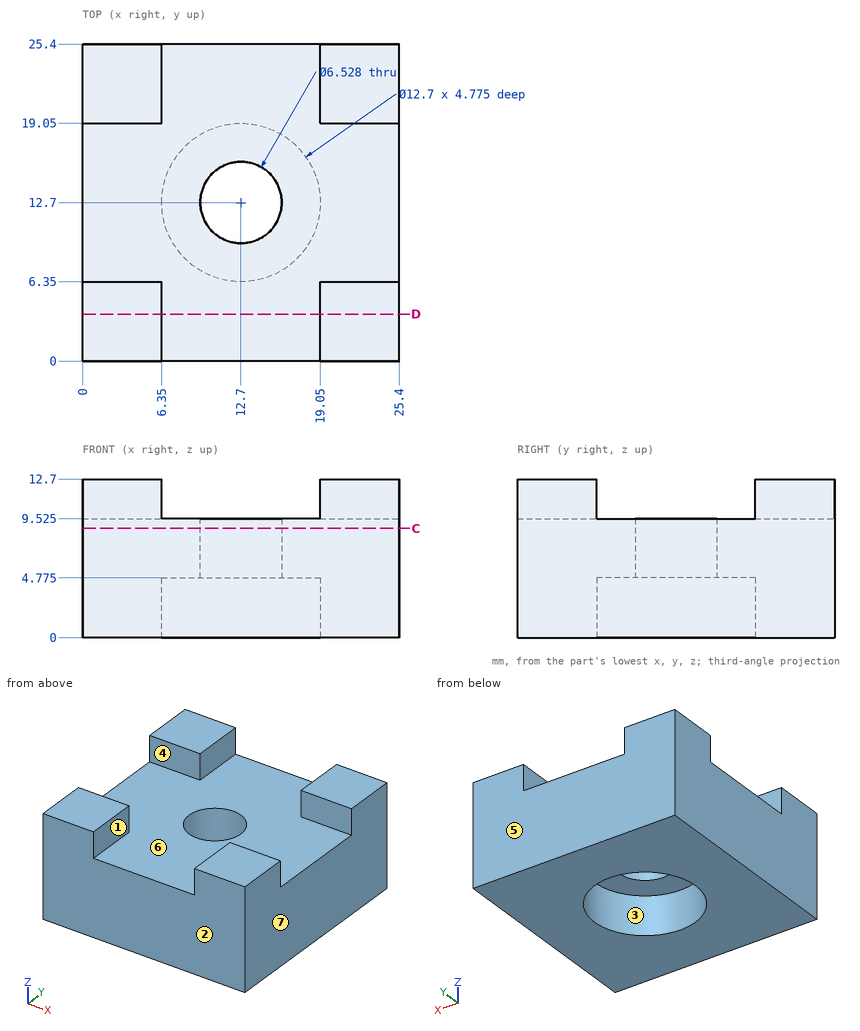
Drawing for the job (mm, zero at the part's lowest x, y, z). A direction names the side the tool comes from. Round coordinates to 2 decimals unless told otherwise and drop trailing zeros. Loops run counter-clockwise (first coordinate to the right, second up) from the corner with the lowest first, then second, coordinate; pieces in that order, holes last. Notation, with made-up numbers: (49.25, -31.5) - (91.25, -31.5) arc R24 cw to (91.25, -2.5) - close; hole circle Ø2 at (44, -10). An arc over 180 degrees is marked (long way). Return JSON: item names as keys, results as strings. Group by question number.
Q1. Tool access for the marked faces 1, 2, 3 and 4: list every direction of +Z, -Z, +X, -X, +Y, -Y with a clear straight run to the whole face (end or side of a thin tool).
Q2. Drill centre lines: line 1 along Y through (x, z) = (12.7, 6.15); line 2 along Y through (x, z) = (12.7, 3.6); line 3 along Z through (x, y) = (16.5, 18.75) (3 decimals). Where is each one in solid material? Low to high. Write a range as [from, to].
Q3. Flat gauge pins, fed straight in: pin 1 Ø7.5 at (x, y) = (12.7, 12.7) entering from +Z (3 decimals); pin 2 Ø4 at (x, y) = (14.5, 12) entering from -Z (3 decimals). Where does each tip first touch, or does it go through?
Q4. Two-plate mould, pull along Y, no slides. Class the marked faces 5, 6 and 7: +Y half, -Y half, draft (parallel to the pull), parting line (faces both ways), or undercut.
Q5. Band-saw the part on D-D on y = 3.75. Give the cut face in (x, z) (3 decimals).
Q6. Band-saw the part on C-C on z = 8.75. Give the cut face in (x, y), plus the area to 3 significant figures.
Solutions:
{
 "1": {"face 1": "+Z, +Y, -Y", "face 2": "+Z, -Z, +X, -X, -Y", "face 3": "-Z", "face 4": "+Z, +X, -X"},
 "2": {"line 1": "y = [0, 9.44], [15.96, 25.4]", "line 2": "y = [0, 6.35], [19.05, 25.4]", "line 3": "z = [0, 9.525]"},
 "3": {"pin 1": "stops at z = 9.525", "pin 2": "stops at z = 4.775"},
 "4": {"face 5": "+Y half", "face 6": "undercut", "face 7": "draft"},
 "5": {"outline": "(0, 0) - (25.4, 0) - (25.4, 12.7) - (19.05, 12.7) - (19.05, 9.525) - (6.35, 9.525) - (6.35, 12.7) - (0, 12.7) - close"},
 "6": {"outline": "(0, 0) - (25.4, 0) - (25.4, 25.4) - (0, 25.4) - close; hole circle Ø6.53 at (12.7, 12.7)", "area": "612 mm^2"}
}
